```python
from build123d import *

# Parameters (mm, degrees)
SKETCH2_W           = 7.62
SKETCH2_H           = 2.54
BOSS_EXTRUDE1_DEPTH = 2.54
SKETCH3_W           = 0.64
SKETCH3_H           = 0.64
CUT_EXTRUDE1_DEPTH  = 5.751904881


with BuildPart() as part:
    # Sketch2 → Boss-Extrude1 (new body)
    with BuildSketch(Plane(origin=(0, 0, 0), x_dir=(1, 0, 0), z_dir=(0, 1, 0))):
        Rectangle(SKETCH2_W, SKETCH2_H)
    extrude(amount=BOSS_EXTRUDE1_DEPTH)

    # Sketch3 → Cut-Extrude1 (cut, through all)
    with BuildSketch(Plane(origin=(0, 2.54, 0), x_dir=(1, 0, 0), z_dir=(0, 1, 0))):
        Rectangle(SKETCH3_W, SKETCH3_H)
        with Locations((-2.54, 0)):
            Rectangle(SKETCH3_W, SKETCH3_H)
        with Locations((2.54, 0)):
            Rectangle(SKETCH3_W, SKETCH3_H)
    extrude(amount=-CUT_EXTRUDE1_DEPTH, mode=Mode.SUBTRACT)


solid = part.part
```
Geometry: final body of the model. Coordinates: model frame, mm. Coordinates: 2 decimals unless noted, no trailing zeros. Write each loop counter-clockwise with the first axis right and the second up, starting at its lowest first coordinate (ties: lowest second). Pieces come first, ordered by that corner, then holes. Notation, with made-up numbers: M 79,38.25 L 88,38.25 A16 cw 88,57.25 Z; hole C 87.25,49.5 d2. An arc over 180 degrees is marked long. Use CSV: the item, a comma, the result in double quotes. Start each with the question number.
1. Cut plane C-C on y = 0.9. Return the cut outline in (x, z), plus the area to 3 significant figures.
2. Cut plane B-B on z = -0.05. Return the cut outline in (x, y).
3. Cut plane A-A on x = 0. Return the cut outline in (y, z).
4. Ray query, probe 1 along X at (y, z) = (1.8, 0.2); probe 2 along Z at (x, y) = (-2.75, 1.95). Return the intervals inside material, ascending.
5. First-contact query: P1, Ø1.5, axis at x = -2, z = 0, coming from the -Y side. Flat tip, straight axial feed; report the tip coordinate or a pass-through.
Entries:
1,outline,"M -3.81,-1.27 L 3.81,-1.27 L 3.81,1.27 L -3.81,1.27 Z; hole M -2.86,-0.32 L -2.22,-0.32 L -2.22,0.32 L -2.86,0.32 Z; hole M -0.32,-0.32 L 0.32,-0.32 L 0.32,0.32 L -0.32,0.32 Z; hole M 2.22,-0.32 L 2.86,-0.32 L 2.86,0.32 L 2.22,0.32 Z"
1,area,"18.1 mm²"
2,outline,"M -3.81,0 L -2.86,0 L -2.86,2.54 L -3.81,2.54 Z; M -2.22,0 L -0.32,0 L -0.32,2.54 L -2.22,2.54 Z; M 0.32,0 L 2.22,0 L 2.22,2.54 L 0.32,2.54 Z; M 2.86,0 L 3.81,0 L 3.81,2.54 L 2.86,2.54 Z"
3,outline,"M 0,-1.27 L 2.54,-1.27 L 2.54,-0.32 L 0,-0.32 Z; M 0,0.32 L 2.54,0.32 L 2.54,1.27 L 0,1.27 Z"
4,probe 1,"-3.81 to -2.86, -2.22 to -0.32, 0.32 to 2.22, 2.86 to 3.81"
4,probe 2,"-1.27 to -0.32, 0.32 to 1.27"
5,P1,"y = 0"
